```python
from build123d import *

# Parameters (mm, degrees)
F1_DEPTH = 2.34
F2_DEPTH = 7.3
F3_R     = 1.5
F4_DEPTH = 4.5


with BuildPart() as f1:
    # F0 (on Top) → F1 (new body)
    with BuildSketch(Plane.XY):
        Polygon((-11.837547, 13.173781), (-4.337547, 13.173781), (-2.337547, 13.173781), (-2.337547, 19.972851), (-11.837547, 19.972851), align=None)
        Polygon((-2.337547, 13.173781), (-0.337547, 13.173781), (7.162453, 13.173781), (7.162453, 19.972851), (-2.337547, 19.972851), align=None)
        Polygon((-4.337547, 13.173781), (-4.337547, 10.173781), (-0.337547, 10.173781), (-0.337547, 13.173781), (-2.337547, 13.173781), align=None)
    extrude(amount=F1_DEPTH)

    # F0 (on Top) → F2 (join)
    with BuildSketch(Plane.XY):
        Polygon((-4.337547, 10.173781), (-9.837547, 10.173781), (-9.837547, 4.423781), (-5.337547, 4.423781), (-5.337547, 1.173781), (-9.837547, 1.173781), (-9.837547, -0.826219), (5.162453, -0.826219), (5.162453, 1.173781), (0.662453, 1.173781), (0.662453, 4.423781), (5.162453, 4.423781), (5.162453, 10.173781), (-0.337547, 10.173781), align=None)
    extrude(amount=F2_DEPTH)

    # F3 (on face) → F4 (join)
    with BuildSketch(Plane(origin=(0, 0, 0), x_dir=(1, 0, 0), z_dir=(0, 0, -1))):
        with Locations((-2.347653, -16.573316)):
            Circle(F3_R)
    extrude(amount=F4_DEPTH)


solid = f1.part
```
The listing builds one solid part. Answer for the finished solid, in the listing's coordinates (mm). A direction names the side the tool comes from. Coordinates: 2 decimals unless noted, no trailing zeros. Order: outer loops, then holes, each group sorted by start corner. A loop starts at its lowest first (then second) coordinate and runs counter-clockwise, first axis right, second up. Notation, with made-up numbers: M 55.25,66.25 L 76.25,66.25 A18 cw 76.25,99.25 Z; hole C 7.5,24.5 d5. An arc over 180 degrees is marked long. Answer as a JSON object with one key per item and string values. Group by question number.
1. Section B-B on z = 5.5 is taken. Write down the section's boundary in (x, y).
2. Section C-C on y = 6 is taken. Write down the section's boundary in (x, z), then the cut area to 4 significant figures.
3. Section D-D on z = 0.5 is taken. Write down the section's boundary in (x, y).
4. Straight lines are drawn through the part: line 1 (Y direction, x = -9.75, z = 1.5); line 2 (Y direction, x = -6.5, z = 6.5); line 3 (X direction, y = 0.25, z = 4.25). For each, find the intervals that lie inside material, in ascending order.
5. Determine the mould class of faces 1 (the flat face through (-2, 17, -4.5)), 2 (the flat face through (-5.338, 3, 4)), 3 (the flat face through (-2, 19.973, 1)) for opening direction Y: released by +Y, released by -Y, zero draft, split by the parting line, or undercut.
6. Flat-ended cylindrical pins translate along their axes: P1, Ø5, axis at x = -3.5, y = 15, coming from the +Z side; P2, Ø2, axis at x = -1.5, z = 3, coming from the +Y side; P3, Ø6.5, axis at y = 6, z = 4.5, coming from the -X side; P4, Ø6, axis at y = 9, z = 5.5, coming from the +X side. Find the tip coordinate at first contact, or state that the pin passes through.
7. Section A-A on x = -6.5 is taken. Write down the section's boundary in (y, z), then the cut area to 3 significant figures.
8. A tool of negligible diameter and unlimited length cuts with its end or side. For faces 4 (the flat face through (-8, 4.424, 4)), 5 (the flat face through (-0.338, 12, 1)), 6 (the flat face through (-2, 16, 2.34)), 7 (the flat face through (-9.838, 7, 4)), from which of +Z, -Z, +X, -X, +Y, -Y can it reach the whole face along a straight path? Write none if from no direction.
Values follow:
{
 "1": {"outline": "M -9.84,-0.83 L 5.16,-0.83 L 5.16,1.17 L 0.66,1.17 L 0.66,4.42 L 5.16,4.42 L 5.16,10.17 L -9.84,10.17 L -9.84,4.42 L -5.34,4.42 L -5.34,1.17 L -9.84,1.17 Z"},
 "2": {"outline": "M -9.84,0 L 5.16,0 L 5.16,7.3 L -9.84,7.3 Z", "area": "109.5 mm2"},
 "3": {"outline": "M -11.84,13.17 L -4.34,13.17 L -4.34,10.17 L -9.84,10.17 L -9.84,4.42 L -5.34,4.42 L -5.34,1.17 L -9.84,1.17 L -9.84,-0.83 L 5.16,-0.83 L 5.16,1.17 L 0.66,1.17 L 0.66,4.42 L 5.16,4.42 L 5.16,10.17 L -0.34,10.17 L -0.34,13.17 L 7.16,13.17 L 7.16,19.97 L -11.84,19.97 Z"},
 "4": {"line 1": "-0.83 to 1.17, 4.42 to 10.17, 13.17 to 19.97", "line 2": "-0.83 to 1.17, 4.42 to 10.17", "line 3": "-9.84 to 5.16"},
 "5": {"face 1": "zero draft", "face 2": "undercut", "face 3": "released by +Y"},
 "6": {"P1": "z = 2.34", "P2": "y = 19.97", "P3": "x = -9.84", "P4": "x = 5.16"},
 "7": {"outline": "M -0.83,0 L 1.17,0 L 1.17,7.3 L -0.83,7.3 Z; M 4.42,0 L 10.17,0 L 10.17,7.3 L 4.42,7.3 Z; M 13.17,0 L 19.97,0 L 19.97,2.34 L 13.17,2.34 Z", "area": "72.5 mm2"},
 "8": {"face 4": "+Z, -Z, -X", "face 5": "+Z, -Z, +X", "face 6": "+Z, +X, -X, +Y", "face 7": "+Z, -Z, -X, -Y"}
}
